Work out the finished part from the listing and answer in its coordinate system (mm). A direction names the side the tool comes from. Coordinates: 2 decimals unless noted, no trailing zeros. Order: outer loops, then holes, each group sorted by start corner. A loop starts at its lowest first (then second) coordinate and runs counter-clockwise, first axis right, second up. Notation, with made-up numbers: (25, 30.25) -> (60, 30.25) arc R10 ccw to (60, 46.25) -> close; hole circle Ø1 at (57, 63.25). An arc over 180 degrees is marked (long way). Write item = value, one per line. Start each with the question number.
Q1. A straight line is drawn through the part: L1, parallel to Y at x = 8, z = -13. Find the intervals that lie inside material, in ascending order. Write a range as from..to.
Q2. The part is cut by section C-C, the plane y = 1.25. Count the separate pieces of the cut face and the enclosed holes in it, plus the area to 3 significant figures.
Q3. The part is cut by section B-B, the plane x = 29.5. Determine the outline of the cut face in (y, z), plus the area to 3 significant figures.
Q4. Flat-ended cylindrical pins translate along their axes: pin 1 (2.5 mm diameter, centred on x = -57, y = 1, fed in from -Z); pin 2 (5 mm diameter, centred on x = -38, z = 9.5, fed in from -Y); pin 3 (3.5 mm diameter, centred on y = 2, z = -31.5, fed in from +X). Find the tip coordinate at first contact, or state that the pin passes through.
Q5. For a pull along X with two mould halves and no side action, classify faces 1 (the cylindrical face through (42.23, -10.85, 31.93)), 2 (the flat face through (-45, -22, -30)), 3 (the flat face through (-30.932, 1, -41)), 4 (the flat face through (-3, 1, 35.048)) as +X half, -X half, draft (parallel to the pull), parting line (faces both ways), or undercut.
Q6. The part is cut by section A-A, the plane y = -14.25. Determine the outline of the cut face in (x, z) (3 decimals), plus the area to 3 significant figures.
Q7. Which of the six approach directions +Z, -Z, +X, -X, +Y, -Y give full straight-line access (tool end or side, diameter ignored) to faces 5 (the flat face through (14.068, 1, -41)), 6 (the flat face through (49, 1, -17.952)), 7 (the flat face through (-50.932, 1, 30)), 8 (the flat face through (-20.932, 1, 40))?
```python
from build123d import *

# Parameters (mm, degrees)
BOSS_EXTRUDE1_DEPTH  = 3
SKETCH2_R            = 3
BOSS_EXTRUDE2_DEPTH  = 22
SKETCH3_R            = 1.775
CUT_EXTRUDE1_DEPTH   = 81.307853189
SKETCH4_R            = 1.05
CUT_EXTRUDE2_DEPTH   = 81.307853189
LPATTERN1_COUNT      = 9
LPATTERN1_PITCH      = 4
LPATTERN1_COUNT_DIR2 = 9
LPATTERN1_PITCH_DIR2 = 4
SKETCH5_R            = 1.775
CUT_EXTRUDE3_DEPTH   = 81.307853189
SKETCH6_R            = 1.775
CUT_EXTRUDE4_DEPTH   = 81.307853189


with BuildPart() as part:
    # Sketch1 → Boss-Extrude1 (new body)
    with BuildSketch(Plane(origin=(0, 0, 0), x_dir=(1, 0, 0), z_dir=(0, 1, 0))):
        Polygon((-50.932204957, 25.952341431), (-50.932204957, 35.952341431), (-30.932204957, 35.952341431), (-30.932204957, 45.952341431), (-20.932204957, 45.952341431), (-20.932204957, 35.952341431), (14.067795043, 35.952341431), (14.067795043, 45.952341431), (24.067795043, 45.952341431), (24.067795043, 35.952341431), (44.067795043, 35.952341431), (44.067795043, 25.952341431), (54.067795043, 25.952341431), (54.067795043, 17.952341431), (44.067795043, 17.952341431), (44.067795043, -17.047658569), (54.067795043, -17.047658569), (54.067795043, -25.047658569), (44.067795043, -25.047658569), (44.067795043, -35.047658569), (24.067795043, -35.047658569), (24.067795043, -45.047658569), (14.067795043, -45.047658569), (14.067795043, -35.047658569), (-20.932204957, -35.047658569), (-20.932204957, -45.047658569), (-30.932204957, -45.047658569), (-30.932204957, -35.047658569), (-50.932204957, -35.047658569), (-50.932204957, -25.047658569), (-60.932204957, -25.047658569), (-60.932204957, -17.047658569), (-50.932204957, -17.047658569), (-50.932204957, 17.952341431), (-60.932204957, 17.952341431), (-60.932204957, 25.952341431), align=None)
    extrude(amount=BOSS_EXTRUDE1_DEPTH)

    # Sketch2 → Boss-Extrude2 (add)
    with BuildSketch(Plane.XZ):
        with Locations(Location((-46.432204957, 30.547658569, 0), (0, 0, 90))):
            Circle(SKETCH2_R)
        with Locations(Location((-46.432204957, -31.452341431, 0), (0, 0, 90))):
            Circle(SKETCH2_R)
        with Locations(Location((39.567795043, -31.452341431, 0), (0, 0, 90))):
            Circle(SKETCH2_R)
        with Locations(Location((39.567795043, 30.547658569, 0), (0, 0, 90))):
            Circle(SKETCH2_R)
    extrude(amount=BOSS_EXTRUDE2_DEPTH)

    # Sketch3 → Cut-Extrude1 (cut, through all)
    with BuildSketch(Plane.XZ.offset(22)):
        with Locations(Location((-46.432204957, 30.547658569, 0), (0, 0, 270))):
            Circle(SKETCH3_R)
        with Locations(Location((-46.432204957, -31.452341431, 0), (0, 0, 270))):
            Circle(SKETCH3_R)
        with Locations(Location((39.567795043, -31.452341431, 0), (0, 0, 270))):
            Circle(SKETCH3_R)
        with Locations(Location((39.567795043, 30.547658569, 0), (0, 0, 270))):
            Circle(SKETCH3_R)
    extrude(amount=-CUT_EXTRUDE1_DEPTH, mode=Mode.SUBTRACT)

    # Sketch4 → Cut-Extrude2 (cut, through all)
    with BuildSketch(Plane(origin=(0, 3, 0), x_dir=(1, 0, 0), z_dir=(0, 1, 0))):
        with Locations(Location((-33.432204957, 23.952341431, 0), (0, 0, 270))):
            Circle(SKETCH4_R)
    cut_extrude2 = extrude(amount=-CUT_EXTRUDE2_DEPTH, mode=Mode.SUBTRACT)

    # LPattern1: Cut-Extrude2 9 × 9
    with Locations(*[(i * LPATTERN1_PITCH, 0, j * LPATTERN1_PITCH_DIR2) for i in range(LPATTERN1_COUNT) for j in range(LPATTERN1_COUNT_DIR2) if (i, j) != (0, 0)]):
        add(cut_extrude2, mode=Mode.SUBTRACT)

    # Sketch5 → Cut-Extrude3 (cut, through all)
    with BuildSketch(Plane(origin=(0, 3, 0), x_dir=(1, 0, 0), z_dir=(0, 1, 0))):
        with Locations(Location((-55.932204957, -21.047658569, 0), (0, 0, 270))):
            Circle(SKETCH5_R)
        with Locations(Location((-55.932204957, 21.952341431, 0), (0, 0, 270))):
            Circle(SKETCH5_R)
        with Locations(Location((49.067795043, 21.952341431, 0), (0, 0, 270))):
            Circle(SKETCH5_R)
        with Locations(Location((49.067795043, -21.047658569, 0), (0, 0, 270))):
            Circle(SKETCH5_R)
    extrude(amount=-CUT_EXTRUDE3_DEPTH, mode=Mode.SUBTRACT)

    # Sketch6 → Cut-Extrude4 (cut, through all)
    with BuildSketch(Plane(origin=(0, 3, 0), x_dir=(1, 0, 0), z_dir=(0, 1, 0))):
        with Locations(Location((-25.932204957, 41.452341431, 0), (0, 0, 270))):
            Circle(SKETCH6_R)
        with Locations(Location((19.067795043, 41.452341431, 0), (0, 0, 270))):
            Circle(SKETCH6_R)
        with Locations(Location((-25.932204957, -40.547658569, 0), (0, 0, 270))):
            Circle(SKETCH6_R)
        with Locations(Location((19.067795043, -40.547658569, 0), (0, 0, 270))):
            Circle(SKETCH6_R)
    extrude(amount=-CUT_EXTRUDE4_DEPTH, mode=Mode.SUBTRACT)


solid = part.part
```
Model answer:
q1.L1 = 0..3
q2.separate_pieces = 1
q2.enclosed_holes = 93
q2.area = 7,070 mm2
q3.outline = (0, -35.95) -> (3, -35.95) -> (3, 35.05) -> (0, 35.05) -> close
q3.area = 213 mm2
q4.pin_1 = -25.95
q4.pin_2 = 0
q4.pin_3 = 44.07
q5.face_1 = undercut
q5.face_2 = draft
q5.face_3 = -X half
q5.face_4 = undercut
q6.outline = circle Ø6 at (-46.432, -31.452); circle Ø6 at (-46.432, 30.548); circle Ø6 at (39.568, -31.452); circle Ø6 at (39.568, 30.548); hole circle Ø3.55 at (-46.432, -31.452); hole circle Ø3.55 at (-46.432, 30.548); hole circle Ø3.55 at (39.568, -31.452); hole circle Ø3.55 at (39.568, 30.548)
q6.area = 73.5 mm2
q7.face_5 = -Z, +Y, -Y
q7.face_6 = +X, +Y, -Y
q7.face_7 = +Z, -X, +Y, -Y
q7.face_8 = +Z, +Y, -Y
